Check sheet for the modelled part. Datum: model origin and axes. Units: mm. A direction names the side the tool comes from. Give positions to 0.01 mm unless a question says otherwise; leave off trailing zeros. Write each loop counter-clockwise with the first axis right and the second up, starting at its lowest first coordinate (ties: lowest second). Pieces come first, ordered by that corner, then holes. Notation, with made-up numbers: (-31.75, 23) -> (15.25, 23) arc R28 cw to (15.25, 52) -> close; hole circle Ø4 at (58.25, 70.5). An arc over 180 degrees is marked (long way). Return JSON: item names as keys, results as strings.
from build123d import *

# Parameters (mm, degrees)
SKETCH2_R           = 55
WHEEL_EXTRUDE_DEPTH = 40
WHEEL_INSET_START   = -15
SKETCH4_R           = 30
WHEEL_INSET_DEPTH   = 15
HUB_INSET_DEPTH     = 25


with BuildPart() as part:
    # Sketch2 → Wheel_Extrude (new body)
    with BuildSketch(Plane(origin=(0, 0, 0), x_dir=(1, 0, 0), z_dir=(0, 1, 0))):
        with Locations(Location((0, 0, 0), (0, 0, 270))):
            Circle(SKETCH2_R)
        with BuildLine():
            Line((2, 29.933259094), (2, 12.338962679))
            ThreePointArc((2, 12.338962679), (4.783542905, 11.548494156), (7.310750621, 10.139177746))
            Line((7.310750621, 10.139177746), (19.751796926, 22.580224051))
            ThreePointArc((19.751796926, 22.580224051), (11.480502971, 27.716385975), (2, 29.933259094))
        make_face(mode=Mode.SUBTRACT)
        with BuildLine():
            Line((-2, 29.933259094), (-2, 12.338962679))
            ThreePointArc((-2, 12.338962679), (-4.783542905, 11.548494156), (-7.310750621, 10.139177746))
            Line((-7.310750621, 10.139177746), (-19.751796926, 22.580224051))
            ThreePointArc((-19.751796926, 22.580224051), (-11.480502971, 27.716385975), (-2, 29.933259094))
        make_face(mode=Mode.SUBTRACT)
        with BuildLine():
            Line((22.580224051, 19.751796926), (10.139177746, 7.310750621))
            ThreePointArc((10.139177746, 7.310750621), (11.548494156, 4.783542905), (12.338962679, 2))
            Line((12.338962679, 2), (29.933259094, 2))
            ThreePointArc((29.933259094, 2), (27.716385975, 11.480502971), (22.580224051, 19.751796926))
        make_face(mode=Mode.SUBTRACT)
        with BuildLine():
            Line((29.933259094, -2), (12.338962679, -2))
            ThreePointArc((12.338962679, -2), (11.548494156, -4.783542905), (10.139177746, -7.310750621))
            Line((10.139177746, -7.310750621), (22.580224051, -19.751796926))
            ThreePointArc((22.580224051, -19.751796926), (27.716385975, -11.480502971), (29.933259094, -2))
        make_face(mode=Mode.SUBTRACT)
        with BuildLine():
            Line((19.751796926, -22.580224051), (7.310750621, -10.139177746))
            ThreePointArc((7.310750621, -10.139177746), (4.783542905, -11.548494156), (2, -12.338962679))
            Line((2, -12.338962679), (2, -29.933259094))
            ThreePointArc((2, -29.933259094), (11.480502971, -27.716385975), (19.751796926, -22.580224051))
        make_face(mode=Mode.SUBTRACT)
        with BuildLine():
            Line((-2, -29.933259094), (-2, -12.338962679))
            ThreePointArc((-2, -12.338962679), (-4.783542905, -11.548494156), (-7.310750621, -10.139177746))
            Line((-7.310750621, -10.139177746), (-19.751796926, -22.580224051))
            ThreePointArc((-19.751796926, -22.580224051), (-11.480502971, -27.716385975), (-2, -29.933259094))
        make_face(mode=Mode.SUBTRACT)
        with BuildLine():
            Line((-22.580224051, -19.751796926), (-10.139177746, -7.310750621))
            ThreePointArc((-10.139177746, -7.310750621), (-11.548494156, -4.783542905), (-12.338962679, -2))
            Line((-12.338962679, -2), (-29.933259094, -2))
            ThreePointArc((-29.933259094, -2), (-27.716385975, -11.480502971), (-22.580224051, -19.751796926))
        make_face(mode=Mode.SUBTRACT)
        with BuildLine():
            Line((-29.933259094, 2), (-12.338962679, 2))
            ThreePointArc((-12.338962679, 2), (-11.548494156, 4.783542905), (-10.139177746, 7.310750621))
            Line((-10.139177746, 7.310750621), (-22.580224051, 19.751796926))
            ThreePointArc((-22.580224051, 19.751796926), (-27.716385975, 11.480502971), (-29.933259094, 2))
        make_face(mode=Mode.SUBTRACT)
    extrude(amount=WHEEL_EXTRUDE_DEPTH)

    # Sketch4 → Wheel_Inset (cut)
    with BuildSketch(Plane(origin=(0, 40, 0), x_dir=(1, 0, 0), z_dir=(0, 1, 0)).offset(WHEEL_INSET_START)):
        with Locations(Location((0, 0, 0), (0, 0, 93.822553729))):
            Circle(SKETCH4_R)
    extrude(amount=WHEEL_INSET_DEPTH, mode=Mode.SUBTRACT)

    # Sketch4_4 → Hub_Inset (cut)
    with BuildSketch(Plane(origin=(0, 40, 0), x_dir=(1, 0, 0), z_dir=(0, 1, 0))):
        Polygon((6.92820323, 0), (3.464101615, 6), (-3.464101615, 6), (-6.92820323, 0), (-3.464101615, -6), (3.464101615, -6), align=None)
    extrude(amount=-HUB_INSET_DEPTH, mode=Mode.SUBTRACT)


solid = part.part
(1) Cross-section at B-B on x = 15.5. Enter the section's corners in (y, z), then the cut area to 3 significant figures.
Reply:
{"outline": "(0, -52.77) -> (40, -52.77) -> (40, -25.69) -> (0, -25.69) -> close; (0, -18.33) -> (25, -18.33) -> (25, -12.67) -> (0, -12.67) -> close; (0, -2) -> (25, -2) -> (25, 2) -> (0, 2) -> close; (0, 12.67) -> (25, 12.67) -> (25, 18.33) -> (0, 18.33) -> close; (0, 25.69) -> (40, 25.69) -> (40, 52.77) -> (0, 52.77) -> close", "area": "2,550 mm^2"}
(2) Release check for a two-part mould opening along Z. For faces 3 (the cylindrical face through (-48.794, 19.72, 25.379)), 4 (the flat face through (1, 0, -1)), 5 (the flat face through (-21, 12, 2)) record: pulls with the +Z half, pulls with the -Z half, needs draft (parallel to the pull), parting line crosses it, or undercut.
Reply:
{"face 3": "parting line crosses it", "face 4": "needs draft", "face 5": "undercut"}
(3) Thickness scan on L1, parallel to Z at x = -23, y = 11.5; L2, parallel to X at y = 3, z = 26; L3, parallel to X at y = 18.5, z = -17. Record the ranges inside material, lowest first.
Reply:
{"L1": "-49.96 to -19.26, -2 to 2, 19.26 to 49.96", "L2": "-48.47 to -14.97, -2 to 2, 14.97 to 48.47", "L3": "-52.31 to -24.72, -19.83 to -14.17, -2 to 2, 14.17 to 19.83, 24.72 to 52.31"}
(4) Cross-section at C-C on y = 27. Enter the section's corners in (x, z), then the cut area to 3 significant figures.
Reply:
{"outline": "circle Ø110 at (0, 0); hole circle Ø60 at (0, 0)", "area": "6,680 mm^2"}
(5) Cross-section at D-D on x = 0. Enter the section's corners in (y, z), then the cut area to 3 significant figures.
Reply:
{"outline": "(0, -55) -> (40, -55) -> (40, -30) -> (25, -30) -> (25, -6) -> (15, -6) -> (15, 6) -> (25, 6) -> (25, 30) -> (40, 30) -> (40, 55) -> (0, 55) -> close", "area": "3,380 mm^2"}
(6) Cross-section at A-A on y = 11.5. State how many separate pieces and enclosed holes the cut face has, then the cut area to 3 significant figures.
Reply:
{"separate pieces": "1", "enclosed holes": "8", "area": "7,730 mm^2"}
(7) Set-up check for faces 1 (the flat face through (16.27, 12.32, 13.44)), 2 (the flat face through (0, 20, -6)): record each of +Z, -Z, +X, -X, +Y, -Y from which the full face is reachable in a straight line by a thin tool's end or side.
Reply:
{"face 1": "+Y, -Y", "face 2": "+Y"}
(8) Depth check by flat-ended pin: pin 1 Ø5.5 at (x, y) = (-23.5, 15.5) entering from +Z; pin 2 Ø19.5 at (y, z) = (18, -17) entering from +X; pin 3 Ø19.5 at (x, y) = (21.5, 17) entering from +Z. Enter the tip coordinate at first touch or a pass-through.
Reply:
{"pin 1": "z = 50.94", "pin 2": "x = 54.52", "pin 3": "z = 53.73"}
